For this review, use the dimensioned drawing (mm, ordinates from the lowest corner) and the shaded views. Round coordinates to 2 decimals unless told otherwise and drop trailing zeros. Write each loop counter-clockwise with the first axis right and the second up, starting at its lowest first coordinate (ties: lowest second). Pieces come first, ordered by that corner, then holes.
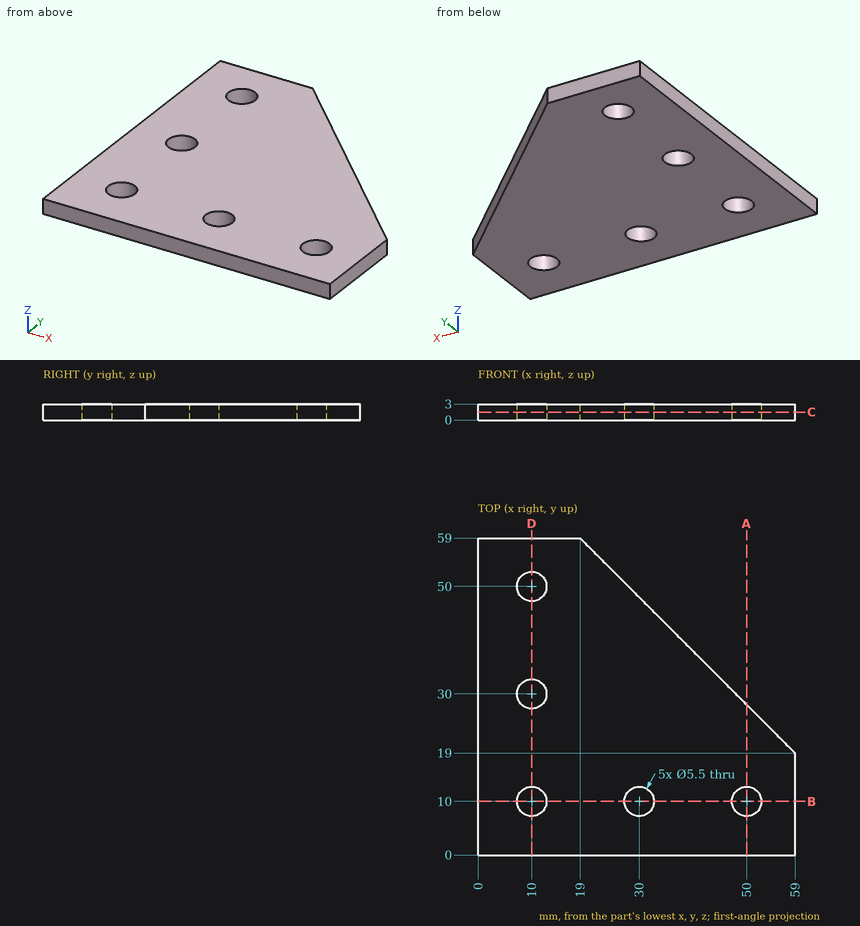
(1) For line 1 along Y through (x, z) = (10, 1.15); line 2 along X through (y, z) = (12, 1.65); line 3 along X through (y, z) = (10.5, 1.85), list the stretches that pass through material, from the lowest coordinate up.
Geometry check:
line 1: y = 0 to 7.25, 12.75 to 27.25, 32.75 to 47.25, 52.75 to 59
line 2: x = 0 to 8.11, 11.89 to 28.11, 31.89 to 48.11, 51.89 to 59
line 3: x = 0 to 7.3, 12.7 to 27.3, 32.7 to 47.3, 52.7 to 59
(2) We need section B-B, the plane y = 10. Give the boundary of the cut face in (x, z).
Geometry check:
outline: (0, 0) - (7.25, 0) - (7.25, 3) - (0, 3) - close; (12.75, 0) - (27.25, 0) - (27.25, 3) - (12.75, 3) - close; (32.75, 0) - (47.25, 0) - (47.25, 3) - (32.75, 3) - close; (52.75, 0) - (59, 0) - (59, 3) - (52.75, 3) - close
(3) We need section A-A, the plane x = 50. Give the boundary of the cut face in (y, z).
Geometry check:
outline: (0, 0) - (7.25, 0) - (7.25, 3) - (0, 3) - close; (12.75, 0) - (28, 0) - (28, 3) - (12.75, 3) - close
(4) We need section C-C, the plane z = 1.5. Give the boundary of the cut face in (x, y), and give its area (3 significant figures).
Geometry check:
outline: (0, 0) - (59, 0) - (59, 19) - (19, 59) - (0, 59) - close; hole circle Ø5.5 at (10, 10); hole circle Ø5.5 at (10, 30); hole circle Ø5.5 at (10, 50); hole circle Ø5.5 at (30, 10); hole circle Ø5.5 at (50, 10)
area: 2,560 mm2
